from build123d import *

# Parameters (mm, degrees)
ESQUISSE1_R        = 4
ESQUISSE1_R_2      = 2.1
BOSS_EXTRU_3_DEPTH = 2
ESQUISSE1_3_R      = 4
ESQUISSE1_3_R_2    = 2.1
BOSS_EXTRU_4_DEPTH = 10


with BuildPart() as part:
    # Esquisse1 → Boss.-Extru.3 (new body)
    # profile 1 of 2: a face of its own
    with BuildSketch(Plane.XY):
        with BuildLine():
            Line((0, 5), (0, 9.5))
            ThreePointArc((0, 9.5), (1.486127418, 9.383039236), (2.935661447, 9.035036905))
            Line((2.935661447, 9.035036905), (1.545084972, 4.755282581))
            ThreePointArc((1.545084972, 4.755282581), (2.269952499, 4.455032621), (2.938926261, 4.045084972))
            Line((2.938926261, 4.045084972), (5.583959897, 7.685661447))
            ThreePointArc((5.583959897, 7.685661447), (6.717514421, 6.717514421), (7.685661447, 5.583959897))
            Line((7.685661447, 5.583959897), (4.045084972, 2.938926261))
            ThreePointArc((4.045084972, 2.938926261), (4.455032621, 2.269952499), (4.755282581, 1.545084972))
            Line((4.755282581, 1.545084972), (9.035036905, 2.935661447))
            ThreePointArc((9.035036905, 2.935661447), (9.383039236, 1.486127418), (9.5, 0))
            Line((9.5, 0), (5, 0))
            ThreePointArc((5, 0), (4.938441703, -0.782172325), (4.755282581, -1.545084972))
            Line((4.755282581, -1.545084972), (9.035036905, -2.935661447))
            ThreePointArc((9.035036905, -2.935661447), (8.46456198, -4.312909748), (7.685661447, -5.583959897))
            Line((7.685661447, -5.583959897), (4.045084972, -2.938926261))
            ThreePointArc((4.045084972, -2.938926261), (3.535533906, -3.535533906), (2.938926261, -4.045084972))
            Line((2.938926261, -4.045084972), (5.583959897, -7.685661447))
            ThreePointArc((5.583959897, -7.685661447), (4.312909748, -8.46456198), (2.935661447, -9.035036905))
            Line((2.935661447, -9.035036905), (1.545084972, -4.755282581))
            ThreePointArc((1.545084972, -4.755282581), (0.782172325, -4.938441703), (0, -5))
            Line((0, -5), (0, -9.5))
            ThreePointArc((0, -9.5), (-1.486127418, -9.383039236), (-2.935661447, -9.035036905))
            Line((-2.935661447, -9.035036905), (-1.545084972, -4.755282581))
            ThreePointArc((-1.545084972, -4.755282581), (-2.269952499, -4.455032621), (-2.938926261, -4.045084972))
            Line((-2.938926261, -4.045084972), (-5.583959897, -7.685661447))
            ThreePointArc((-5.583959897, -7.685661447), (-6.717514421, -6.717514421), (-7.685661447, -5.583959897))
            Line((-7.685661447, -5.583959897), (-4.045084972, -2.938926261))
            ThreePointArc((-4.045084972, -2.938926261), (-4.455032621, -2.269952499), (-4.755282581, -1.545084972))
            Line((-4.755282581, -1.545084972), (-9.035036905, -2.935661447))
            ThreePointArc((-9.035036905, -2.935661447), (-9.383039236, -1.486127418), (-9.5, 0))
            Line((-9.5, 0), (-5, 0))
            ThreePointArc((-5, 0), (-4.938441703, 0.782172325), (-4.755282581, 1.545084972))
            Line((-4.755282581, 1.545084972), (-9.035036905, 2.935661447))
            ThreePointArc((-9.035036905, 2.935661447), (-8.46456198, 4.312909748), (-7.685661447, 5.583959897))
            Line((-7.685661447, 5.583959897), (-4.045084972, 2.938926261))
            ThreePointArc((-4.045084972, 2.938926261), (-3.535533906, 3.535533906), (-2.938926261, 4.045084972))
            Line((-2.938926261, 4.045084972), (-5.583959897, 7.685661447))
            ThreePointArc((-5.583959897, 7.685661447), (-4.312909748, 8.46456198), (-2.935661447, 9.035036905))
            Line((-2.935661447, 9.035036905), (-1.545084972, 4.755282581))
            ThreePointArc((-1.545084972, 4.755282581), (-0.782172325, 4.938441703), (0, 5))
        make_face()
        Circle(ESQUISSE1_R, mode=Mode.SUBTRACT)
    # profile 2 of 2: a face of its own
    with BuildSketch(Plane.XY):
        Circle(ESQUISSE1_R)
        Circle(ESQUISSE1_R_2, mode=Mode.SUBTRACT)
    extrude(amount=BOSS_EXTRU_3_DEPTH)

    # Esquisse1_3 → Boss.-Extru.4 (add)
    with BuildSketch(Plane.XY):
        Circle(ESQUISSE1_3_R)
        Circle(ESQUISSE1_3_R_2, mode=Mode.SUBTRACT)
    extrude(amount=BOSS_EXTRU_4_DEPTH)


solid = part.part
Design review of the part built by this model. Coordinates are the model's own, in mm. A direction names the side the tool comes from. Give positions to 0.01 mm unless a question says otherwise; leave off trailing zeros. Loops run counter-clockwise (first coordinate to the right, second up) from the corner with the lowest first, then second, coordinate; pieces in that order, holes last. Notation, with made-up numbers: (73.25, -7.5) -> (92.25, -7.5) arc R28 cw to (92.25, 26.5) -> close; hole circle Ø9 at (14, 14.5). An arc over 180 degrees is marked (long way). One line per question, with ' | ' between items. Start each with the question number.
(1) For faces 1 (the face through (-0.793, 4.937, 0.986)), 2 (the face through (-6.865, 2.231, 0.986)), 3 (the face through (4.94, -0.77, 0.99)), 4 (the face through (3.54, -3.53, 0.99)), 5 (the face through (2.25, -6.93, 0.99)), list the 3-axis set-ups (+Z, -Z, +X, -X, +Y, -Y) from which the entire face can be reached by the end or side of a thin tool; tool diameter is ignored.
(2) For line 1 (Y direction, x = 0, z = 5.5); line 2 (Z direction, x = -3.5, y = -4); line 3 (X direction, y = 1, z = 7), list the stretches that pass through material, from the lowest coordinate up.
(3) Insertion check: P1, Ø2, axis at y = 2, z = 7, coming from the -X side; P2, Ø2, axis at y = 6.5, z = 1, coming from the -X side; P3, Ø5, axis at x = -6, y = 3.5, coming from the +Z side. Each pin has a flat end and moves straight along its axis. Give the tip position at first contact, or say it passes through.
(4) We need section C-C (x = 7). State the section outline as (y, z) points, and give its area (3 significant figures).
(5) Draft analysis for pull direction Y (two halves, no side actions). For faces 6 (the face through (2.003, 0.631, 4.93)), 7 (the face through (-4.45, -2.28, 0.99)), 8 (the face through (-0.867, -3.905, 5.944)), 9 (the face through (4.332, -8.455, 0.986)), state which applies: +Y half, -Y half, draft (parallel to the pull), parting line (faces both ways), or undercut.
(6) We need section D-D (y = -6.75). State the section outline as (x, z) points, and give its area (3 significant figures).
(7) We need section B-B (y = 3.25). State the section outline as (x, z) points.
(8) We need section A-A (x = 0.5). State the section outline as (y, z) points.
The answers:
1) face 1: +Z, -Z, +Y | face 2: +Z, -Z, -X | face 3: +Z, -Z, +X | face 4: +Z, -Z | face 5: +Z, -Z, -Y
2) line 1: y = -4 to -2.1, 2.1 to 4 | line 2: z = 0 to 2 | line 3: x = -3.87 to -1.85, 1.85 to 3.87
3) P1: stops at x = -3.87 | P2: stops at x = -7.75 | P3: stops at z = 2
4) outline: (-5.09, 0) -> (-2.27, 0) -> (-2.27, 2) -> (-5.09, 2) -> close; (0, 0) -> (2.27, 0) -> (2.27, 2) -> (0, 2) -> close; (5.09, 0) -> (6.42, 0) -> (6.42, 2) -> (5.09, 2) -> close | area: 12.8 mm^2
5) face 6: undercut | face 7: undercut | face 8: parting line | face 9: -Y half
6) outline: (-6.68, 0) -> (-4.9, 0) -> (-4.9, 2) -> (-6.68, 2) -> close; (-2.19, 0) -> (0, 0) -> (0, 2) -> (-2.19, 2) -> close; (2.19, 0) -> (4.9, 0) -> (4.9, 2) -> (2.19, 2) -> close | area: 13.4 mm^2
7) outline: (-8.93, 0) -> (-4.47, 0) -> (-4.47, 2) -> (-8.93, 2) -> close; (-3.8, 0) -> (4.47, 0) -> (4.47, 2) -> (2.33, 2) -> (2.33, 10) -> (-2.33, 10) -> (-2.33, 2) -> (-3.8, 2) -> close
8) outline: (-4.97, 0) -> (-2.04, 0) -> (-2.04, 10) -> (-3.97, 10) -> (-3.97, 2) -> (-4.97, 2) -> close; (2.04, 0) -> (9.49, 0) -> (9.49, 2) -> (3.97, 2) -> (3.97, 10) -> (2.04, 10) -> close
